Study the drawing (mm; zero at the part's minimum x, y, z) and answer. Coordinates: 2 decimals unless noted, no trailing zeros. Loops run counter-clockwise (first coordinate to the right, second up) from the corner with the lowest first, then second, coordinate; pieces in that order, holes last. Notation, with made-up numbers: (79.25, -30.5) -> (115.25, -30.5) arc R25 ccw to (115.25, 3.5) -> close; hole circle Ø6 at (-31.75, 36.5). An arc over 180 degrees is marked (long way). Answer as a JSON object with one key per item and string values. Group by question number.
Q1. The part is cut by section D-D on x = 26.5. Write down the section's boundary in (y, z).
Q2. Straight lines are drawn through the part: line 1 along Y through (x, z) = (26.5, 2.2); line 2 along Y through (x, z) = (40, 2.5); line 3 along Y through (x, z) = (29, 3.35). For each, find the intervals that lie inside material, in ascending order. Write a range as [from, to].
Q3. The part is cut by section A-A on y = 69. Write down the section's boundary in (x, z), and give its area (3 significant figures).
Q4. The part is cut by section B-B on z = 0.95. Write down the section's boundary in (x, y), and give its area (3 significant figures).
Q5. The part is cut by section C-C on x = 40. Write down the section's boundary in (y, z).
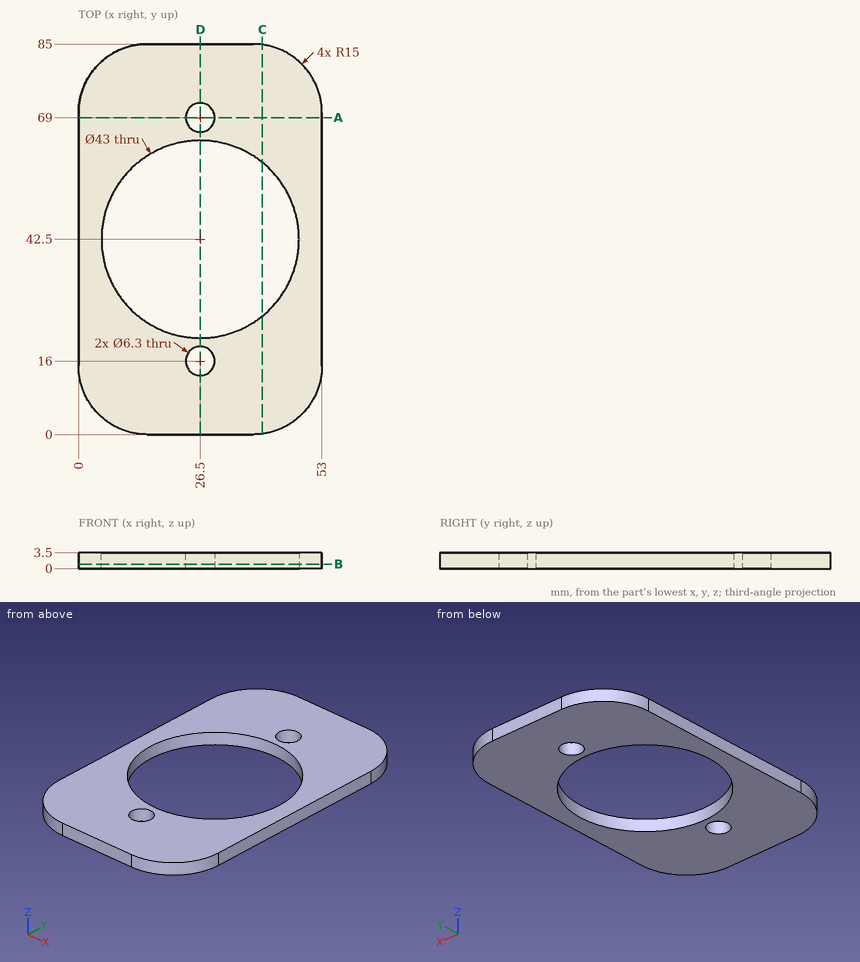
Final values:
{
 "1": {"outline": "(0, 0) -> (12.85, 0) -> (12.85, 3.5) -> (0, 3.5) -> close; (19.15, 0) -> (21, 0) -> (21, 3.5) -> (19.15, 3.5) -> close; (64, 0) -> (65.85, 0) -> (65.85, 3.5) -> (64, 3.5) -> close; (72.15, 0) -> (85, 0) -> (85, 3.5) -> (72.15, 3.5) -> close"},
 "2": {"line 1": "y = [0, 12.85], [19.15, 21], [64, 65.85], [72.15, 85]", "line 2": "y = [0.13, 25.77], [59.23, 84.87]", "line 3": "y = [0, 14.08], [17.92, 21.15], [63.85, 67.08], [70.92, 85]"},
 "3": {"outline": "(0, 0) -> (23.35, 0) -> (23.35, 3.5) -> (0, 3.5) -> close; (29.65, 0) -> (53, 0) -> (53, 3.5) -> (29.65, 3.5) -> close", "area": "163 mm2"},
 "4": {"outline": "(0, 15) arc R15 ccw to (15, 0) -> (38, 0) arc R15 ccw to (53, 15) -> (53, 70) arc R15 ccw to (38, 85) -> (15, 85) arc R15 ccw to (0, 70) -> close; hole circle Ø43 at (26.5, 42.5); hole circle Ø6.3 at (26.5, 16); hole circle Ø6.3 at (26.5, 69)", "area": "2,800 mm2"},
 "5": {"outline": "(0.13, 0) -> (25.77, 0) -> (25.77, 3.5) -> (0.13, 3.5) -> close; (59.23, 0) -> (84.87, 0) -> (84.87, 3.5) -> (59.23, 3.5) -> close"}
}
